```python
from build123d import *

# Parameters (mm, degrees)
SKETCH1_R                = 26
SKETCH1_R_2              = 12.5
BASE_EXTRUDE_DEPTH       = 15
RACCORDO1_R              = 0.5
SCHIZZO1_R               = 25.5
SCHIZZO1_R_2             = 13
TAGLIO_ESTRUSIONE1_DEPTH = 0.1
TAGLIO_ESTRUSIONE2_START = -0.1
SCHIZZO2_R               = 25.5
SCHIZZO2_R_2             = 13
TAGLIO_ESTRUSIONE2_DEPTH = 0.1


with BuildPart() as part:
    # Sketch1 → Base-Extrude (new body)
    with BuildSketch(Plane(origin=(0, 0, 0), x_dir=(0, 0, -1), z_dir=(1, 0, 0))):
        Circle(SKETCH1_R)
        Circle(SKETCH1_R_2, mode=Mode.SUBTRACT)
    extrude(amount=BASE_EXTRUDE_DEPTH)

    # Raccordo1
    raccordo1_edges = [part.edges().sort_by_distance(p)[0] for p in [
        (0, 0, 26),
        (15, 0, 26),
        (0, 0, 12.5),
        (15, 0, 12.5),
    ]]
    fillet(raccordo1_edges, radius=RACCORDO1_R)

    # Schizzo1 → Taglio-Estrusione1 (cut)
    with BuildSketch(Plane.ZY):
        Circle(SCHIZZO1_R)
        Circle(SCHIZZO1_R_2, mode=Mode.SUBTRACT)
    extrude(amount=-TAGLIO_ESTRUSIONE1_DEPTH, mode=Mode.SUBTRACT)

    # Schizzo2 → Taglio-Estrusione2 (cut)
    with BuildSketch(Plane(origin=(15, 0, 0), x_dir=(0, 0, -1), z_dir=(1, 0, 0)).offset(TAGLIO_ESTRUSIONE2_START)):
        with Locations(Location((0, 0, 0), (0, 0, 180))):
            Circle(SCHIZZO2_R)
        with Locations(Location((0, 0, 0), (0, 0, 180))):
            Circle(SCHIZZO2_R_2, mode=Mode.SUBTRACT)
    extrude(amount=TAGLIO_ESTRUSIONE2_DEPTH, mode=Mode.SUBTRACT)


solid = part.part
```
Design review of the part built by this model. Coordinates are the model's own, in mm. Give positions to 0.01 mm unless a question says otherwise; leave off trailing zeros. Order: outer loops, then holes, each group sorted by start corner. A loop starts at its lowest first (then second) coordinate and runs counter-clockwise, first axis right, second up. Notation, with made-up numbers: M 77.25,16 L 88.25,16 A24 cw 88.25,48 Z; hole C 11,0.5 d10. An arc over 180 degrees is marked long. One line per question, with ' | ' between items. Start each with the question number.
Q1. For pin 1 Ø3 at (y, z) = (-12.5, -19.5) entering from +X; pin 2 Ø6 at (x, y) = (3, 16) entering from -Z; pin 3 Ø3 at (x, z) = (13, 4.5) entering from +Y, all flat-tipped, find the tip position at first contact; note any pin that passes through.
Q2. We need section A-A (y = 0). Write out the cut boundary in (x, z), plus the area to 3 significant figures.
Q3. For L1, parallel to Y at x = 7, z = 0; L2, parallel to X at y = -6, z = 23; L3, parallel to Y at x = 2.5, z = 3.5, list the stretches that pass through material, from the lowest coordinate up. Write a range as [from, to].
Q4. We need section C-C (x = 13.5). Write out the cut boundary in (y, z).
Q5. The part is to be moulded in two halves that separate along Y. For faces 1 (the face through (7.402, -15.821, 20.633)), 2 (the face through (7.402, 3.755, -11.923)), 3 (the face through (0.1, 6, -12)), say which applies: +Y half, -Y half, draft (parallel to the pull), parting line (faces both ways), or undercut.
Returned:
1) pin 1: x = 14.9 | pin 2: z = -22.52 | pin 3: y = 25.83
2) outline: M 0,-25.5 A0.5 ccw 0.5,-26 L 14.5,-26 A0.5 ccw 15,-25.5 L 14.9,-25.5 L 14.9,-13 L 15,-13 A0.5 ccw 14.5,-12.5 L 0.5,-12.5 A0.5 ccw 0,-13 L 0.1,-13 L 0.1,-25.5 Z; M 0,13 A0.5 ccw 0.5,12.5 L 14.5,12.5 A0.5 ccw 15,13 L 14.9,13 L 14.9,25.5 L 15,25.5 A0.5 ccw 14.5,26 L 0.5,26 A0.5 ccw 0,25.5 L 0.1,25.5 L 0.1,13 Z | area: 400 mm2
3) L1: [-26, -12.5], [12.5, 26] | L2: [0.1, 14.9] | L3: [-25.76, -12], [12, 25.76]
4) outline: C 0,0 d52; hole C 0,0 d25
5) face 1: parting line | face 2: undercut | face 3: undercut
